Input: part model. Units: mm. Frame: model coordinates. A direction names the side the tool comes from. Round coordinates to 2 decimals unless told otherwise and drop trailing zeros. Loops run counter-clockwise (first coordinate to the right, second up) from the corner with the lowest first, then second, coordinate; pieces in that order, holes last. Notation, with made-up numbers: M 74,42.5 L 78,42.5 A14 ccw 78,57.5 Z; hole C 27.25,14 d11. An arc over 180 degrees is marked long. Return JSON: item names as keys, results as strings. Group by question number.
1) Access query for faces 1 (the face through (-952, 9.516, 432)), 2 (the face through (-917.503, 13, 463)), 3 (the face through (-942.353, 6, 447)). Directions: +Z, -Z, +X, -X, +Y, -Y. A direction counts if a zero-diameter tool reaches every point of the face in a straight line with its end or side. Return the directions, or none.
2) Section B-B (y = -2). Count the separate pieces of the cut face and the enclosed holes in it, plus the area to 3 significant figures.
3) Section C-C (z = 463). Output: boundary loops of the cut face in (x, y), plus the area to 3 significant figures.
4) Material intervals for line 1 (X direction, y = 16.25, z = 447.5); line 2 (Z direction, x = -938, y = 14.75); line 3 (X direction, y = 14.5, z = 450), sorted ascending. Write a range as from..to.
5) Mould query, pull axis Y, two halves, no side actions, for faces 4 (the face through (-950.4, 18.266, 444.1)), 5 (the face through (-931.347, 2.527, 465.554)), 6 (the face through (-925.641, 5.591, 442.045)). Classes: +Y half, -Y half, draft (parallel to the pull), parting line (faces both ways), or undercut.
6) Contact query for flat-ended pins moving along their axis: P1, Ø6, axis at y = 15, z = 460.5, coming from the -X side; P2, Ø9, axis at x = -923, z = 447, coming from the -Y side. Output: stop coordinate, or through.
7) Section A-A (x = -945.5). Output: boundary loops of the cut face in (y, z), plus the area to 3 significant figures.
8) Section D-D (y = 19.25). Output: boundary loops of the cut face in (x, z), plus the area to 3 significant figures.
from build123d import *

# Parameters (mm, degrees)
SKETCH1_W            = 45
SKETCH1_H            = 40
BOSS_EXTRUDE1_DEPTH  = 30
CUT_EXTRUDE1_DEPTH   = 25
SKETCH3_R            = 2
CUT_EXTRUDE2_DEPTH   = 959.969914124
SKETCH7_R            = 2
CUT_EXTRUDE4_DEPTH   = 470.526936912
SKETCH9_W            = 2.7
SKETCH9_H            = 7.5
CUT_EXTRUDE5_DEPTH   = 10.75
CUT_EXTRUDE6_START   = -40
SKETCH9_2_W          = 2.7
SKETCH9_2_H          = 7.5
CUT_EXTRUDE6_DEPTH   = 10.75
SKETCH10_R           = 3.5
CUT_EXTRUDE9_DEPTH   = 1066.96024555
SKETCH13_R           = 4.2
CUT_EXTRUDE10_DEPTH  = 959.969914124
SKETCH14_OUTSIDE_W   = 60.454
SKETCH14_OUTSIDE_H   = 45.454
SKETCH14_OUTSIDE_W_2 = 43
SKETCH14_OUTSIDE_H_2 = 30
CUT_EXTRUDE11_DEPTH  = 959.969914124
FILLET1_R            = 2
SKETCH15_W           = 14
SKETCH15_H           = 7
CUT_EXTRUDE12_DEPTH  = 10
CUT_EXTRUDE13_DEPTH  = 7


with BuildPart() as part:
    # Sketch1 → Boss-Extrude1 (new body)
    with BuildSketch(Plane.XZ.offset(-23.265807416)):
        with Locations((-935.352806229, 446.786082367)):
            Rectangle(SKETCH1_W, SKETCH1_H)
    extrude(amount=BOSS_EXTRUDE1_DEPTH)

    # Sketch2 → Cut-Extrude1 (cut)
    with BuildSketch(Plane.XZ.offset(6.734192584)):
        Polygon((-922.852806229, 453.136935328), (-928.352806229, 449.961508847), (-928.352806229, 443.610655886), (-922.852806229, 440.435229406), (-917.352806229, 443.610655886), (-917.352806229, 449.961508847), align=None)
        Polygon((-947.852806229, 453.136935328), (-953.352806229, 449.961508847), (-953.352806229, 443.610655886), (-947.852806229, 440.435229406), (-942.352806229, 443.610655886), (-942.352806229, 449.961508847), align=None)
    extrude(amount=-CUT_EXTRUDE1_DEPTH, mode=Mode.SUBTRACT)

    # Sketch3 → Cut-Extrude2 (cut, through all)
    with BuildSketch(Plane(origin=(0, 0, 426.786082367), x_dir=(-1, 0, 0), z_dir=(0, 0, -1))):
        with Locations((935.352806229, 1.265807416)):
            Circle(SKETCH3_R)
    extrude(amount=-CUT_EXTRUDE2_DEPTH, mode=Mode.SUBTRACT)

    # Sketch7 → Cut-Extrude4 (cut, through all)
    with BuildSketch(Plane.ZY.offset(957.852806229)):
        with Locations((433.786082367, 13.265807416)):
            Circle(SKETCH7_R)
        with Locations((459.786082367, 13.265807416)):
            Circle(SKETCH7_R)
    extrude(amount=-CUT_EXTRUDE4_DEPTH, mode=Mode.SUBTRACT)

    # Sketch9 → Cut-Extrude5 (cut)
    with BuildSketch(Plane(origin=(0, 0, 426.786082367), x_dir=(-1, 0, 0), z_dir=(0, 0, -1))):
        with Locations((918.852806229, 13.265807416)):
            Rectangle(SKETCH9_W, SKETCH9_H)
        with Locations((951.852806229, 13.265807416)):
            Rectangle(SKETCH9_W, SKETCH9_H)
    extrude(amount=-CUT_EXTRUDE5_DEPTH, mode=Mode.SUBTRACT)

    # Sketch9<2> → Cut-Extrude6 (cut)
    with BuildSketch(Plane(origin=(0, 0, 426.786082367), x_dir=(-1, 0, 0), z_dir=(0, 0, -1)).offset(CUT_EXTRUDE6_START)):
        with Locations((918.852806229, 13.265807416)):
            Rectangle(SKETCH9_2_W, SKETCH9_2_H)
        with Locations((951.852806229, 13.265807416)):
            Rectangle(SKETCH9_2_W, SKETCH9_2_H)
    extrude(amount=CUT_EXTRUDE6_DEPTH, mode=Mode.SUBTRACT)

    # Sketch10 → Cut-Extrude9 (cut, through all)
    with BuildSketch(Plane.XZ.offset(6.734192584)):
        with Locations(Location((-947.852806229, 446.786082367, 0), (0, 0, 270))):
            Circle(SKETCH10_R)
        with Locations(Location((-922.852806229, 446.786082367, 0), (0, 0, 270))):
            Circle(SKETCH10_R)
    extrude(amount=-CUT_EXTRUDE9_DEPTH, mode=Mode.SUBTRACT)

    # Sketch13 → Cut-Extrude10 (cut, through all)
    with BuildSketch(Plane.XY.offset(466.786082367)):
        with Locations((-935.352806229, 1.265807416)):
            Circle(SKETCH13_R)
    extrude(amount=-CUT_EXTRUDE10_DEPTH, mode=Mode.SUBTRACT)

    # Sketch14 outside → Cut-Extrude11 (cut, through all)
    with BuildSketch(Plane(origin=(0, 0, 426.786082367), x_dir=(-1, 0, 0), z_dir=(0, 0, -1))):
        with Locations((935.353, 8.266)):
            Rectangle(SKETCH14_OUTSIDE_W, SKETCH14_OUTSIDE_H)
        with Locations((935.352806229, 8.265807416)):
            Rectangle(SKETCH14_OUTSIDE_W_2, SKETCH14_OUTSIDE_H_2, mode=Mode.SUBTRACT)
    extrude(amount=-CUT_EXTRUDE11_DEPTH, mode=Mode.SUBTRACT)

    # Fillet1
    fillet1_edges = [part.edges().sort_by_distance(p)[0] for p in [
        (-956.852806229, 8.265807416, 466.786082367),
        (-956.852806229, 8.265807416, 426.786082367),
        (-913.852806229, 8.265807416, 426.786082367),
        (-913.852806229, 8.265807416, 466.786082367),
    ]]
    fillet(fillet1_edges, radius=FILLET1_R)

    # Sketch15 → Cut-Extrude12 (cut)
    with BuildSketch(Plane.XZ.offset(6.734192584)):
        with Locations((-935.352806229, 460.786082367)):
            Rectangle(SKETCH15_W, SKETCH15_H)
    extrude(amount=-CUT_EXTRUDE12_DEPTH, mode=Mode.SUBTRACT)

    # Sketch16 → Cut-Extrude13 (cut)
    with BuildSketch(Plane.XY.offset(457.286082367)):
        Polygon((-928.352806229, 5.3072593), (-935.352806229, 9.348711184), (-942.352806229, 5.3072593), (-942.352806229, -2.775644469), (-935.352806229, -6.817096353), (-928.352806229, -2.775644469), align=None)
    extrude(amount=CUT_EXTRUDE13_DEPTH, mode=Mode.SUBTRACT)


solid = part.part
Returned:
{
 "1": {"face 1": "-Z", "face 2": "+Z", "face 3": "-Y"},
 "2": {"separate pieces": "2", "enclosed holes": "2", "area": "1,230 mm^2"},
 "3": {"outline": "M -956.85,-6.73 L -942.35,-6.73 L -942.35,5.31 L -935.35,9.35 L -928.35,5.31 L -928.35,-6.73 L -913.85,-6.73 L -913.85,23.27 L -956.85,23.27 Z; hole M -953.2,9.52 L -950.5,9.52 L -950.5,17.02 L -953.2,17.02 Z; hole M -920.2,9.52 L -917.5,9.52 L -917.5,17.02 L -920.2,17.02 Z", "area": "1,050 mm^2"},
 "4": {"line 1": "x = -956.85..-953.35, -942.35..-928.35, -917.35..-913.85", "line 2": "z = 426.79..432.45, 435.13..458.45, 461.13..466.79", "line 3": "x = -956.85..-953.29, -942.42..-928.29, -917.42..-913.85"},
 "5": {"face 4": "-Y half", "face 5": "undercut", "face 6": "draft"},
 "6": {"P1": "stops at x = -956.85", "P2": "stops at y = 18.27"},
 "7": {"outline": "M -6.73,426.79 L 23.27,426.79 L 23.27,444.19 L 18.27,444.19 L 18.27,441.79 L -6.73,441.79 Z; M -6.73,451.78 L 18.27,451.78 L 18.27,449.38 L 23.27,449.38 L 23.27,466.79 L -6.73,466.79 Z; hole C 13.27,433.79 d4; hole C 13.27,459.79 d4", "area": "899 mm^2"},
 "8": {"outline": "M -956.85,428.79 A2 ccw -954.85,426.79 L -915.85,426.79 A2 ccw -913.85,428.79 L -913.85,464.79 A2 ccw -915.85,466.79 L -954.85,466.79 A2 ccw -956.85,464.79 Z; hole C -947.85,446.79 d7; hole C -922.85,446.79 d7", "area": "1,640 mm^2"}
}
